For this review, take the finished solid that the model builds, in its own axes (mm). A direction names the side the tool comes from. Coordinates: 2 decimals unless noted, no trailing zeros. Loops run counter-clockwise (first coordinate to the right, second up) from the corner with the lowest first, then second, coordinate; pieces in that order, holes last. Notation, with made-up numbers: (-30.5, 85.5) - (5.5, 85.5) arc R12 cw to (5.5, 101.5) - close; hole circle Ø5 at (63.25, 76). An arc over 180 degrees is marked (long way). One line per item, written item: value. Start each with the question number.
1. Take a section at A-A, the plane z = -383. State the section outline as (x, y) points.
2. Insertion check: pin 1 (3 mm diameter, centred on x = -87, z = 12.5, fed in from +Y); pin 2 (18 mm diameter, centred on y = 21, z = -252.34, fed in from -X); pin 3 (4.5 mm diameter, centred on x = 250, z = 221, fed in from -Y); pin 4 (10 mm diameter, centred on x = 521.5, z = 56.5, fed in from -Y). Each pin has a flat end and moves straight along its axis. Give the tip position at first contact, or say it passes through.
3. The part is to be moulded in two halves that separate along X. For faces 1 (the face through (1351.312, 25, -147)), 2 (the face through (1347.312, 25, -147)), 3 (the face through (385, 25, 222.656)), 4 (the face through (-554.688, 25, -157)), say which applies: released by +X, released by -X, zero draft, split by the parting line, or undercut.
4. To check wall thickness, follow line 1 (Z direction, x = -553.3, y = 21); line 2 (X direction, y = 39, z = -11.5); line 3 (Y direction, x = -222.5, z = -376.5). State the ranges of each line that lie inside material, in increasing order. Write a range as from..to.
5. Take a section at B-B, the plane x = 1007. State the section outline as (y, z) points.
6. For faces 5 (the face through (385, -34, -527.344)), 6 (the face through (-550.688, 25, -157)), 7 (the face through (385, -4, -157)), list the 3-axis set-ups (+Z, -Z, +X, -X, +Y, -Y) from which the entire face can be reached by the end or side of a thin tool; tool diameter is ignored.
```python
from build123d import *

# Parameters (mm, degrees)
SKETCH1_W                    = 1906
SKETCH1_H                    = 750
BASE_FLANGE1_DEPTH           = 4
EDGE_FLANGE1_STRIP_W         = 24
EDGE_FLANGE1_STRIP_H         = 4
EDGE_FLANGE1_STRIP_CUT_DEPTH = 1906
EDGE_FLANGE1_DEPTH           = 1906
EDGE_FLANGE2_STRIP_W         = 24
EDGE_FLANGE2_STRIP_H         = 4
EDGE_FLANGE2_STRIP_CUT_DEPTH = 1906
EDGE_FLANGE2_DEPTH           = 1906
EDGE_FLANGE3_STRIP_W         = 24
EDGE_FLANGE3_STRIP_H         = 4
EDGE_FLANGE3_STRIP_CUT_DEPTH = 734
EDGE_FLANGE3_DEPTH           = 734
EDGE_FLANGE4_STRIP_W         = 24
EDGE_FLANGE4_STRIP_H         = 4
EDGE_FLANGE4_STRIP_CUT_DEPTH = 734
EDGE_FLANGE4_DEPTH           = 734
SKETCH18_R                   = 7
CUT_EXTRUDE4_DEPTH           = 1979.516472174
LPATTERN1_COUNT              = 4
LPATTERN1_PITCH              = 200
CUT_EXTRUDE5_DEPTH           = 10
LPATTERN2_COUNT              = 6
LPATTERN2_PITCH              = 300
CUT_EXTRUDE6_DEPTH           = 1545.720516034
LPATTERN3_COUNT              = 6
LPATTERN3_PITCH              = 300


# Sheet-metal steps are written as plain solids
with BuildPart() as part:
    # Sketch1 → Base-Flange1 (new body)
    with BuildSketch(Plane(origin=(0, 0, 0), x_dir=(1, 0, 0), z_dir=(0, 1, 0))):
        with Locations((398.3125, 152.34375)):
            Rectangle(SKETCH1_W, SKETCH1_H)
    extrude(amount=-BASE_FLANGE1_DEPTH)

    # Edge-Flange1 strip (across the edge) → Edge-Flange1 strip cut (cut)
    with BuildSketch(Plane(origin=(-554.6875, -4, -527.34375), x_dir=(0, 0, 1), z_dir=(1, 0, 0))):
        with Locations((-4, -2)):
            Rectangle(EDGE_FLANGE1_STRIP_W, EDGE_FLANGE1_STRIP_H)
    extrude(amount=EDGE_FLANGE1_STRIP_CUT_DEPTH, mode=Mode.SUBTRACT)

    # Edge-Flange1 section (across the edge) → Edge-Flange1 (add)
    with BuildSketch(Plane(origin=(-554.6875, -4, -527.34375), x_dir=(0, 0, 1), z_dir=(1, 0, 0))):
        with BuildLine():
            Line((0, 4), (0, 56))
            Line((0, 56), (4, 56))
            Line((4, 56), (4, 4))
            ThreePointArc((4, 4), (5.171572875, 1.171572875), (8, 0))
            Line((8, 0), (8, -4))
            ThreePointArc((8, -4), (2.343145751, -1.656854249), (0, 4))
        make_face()
    extrude(amount=EDGE_FLANGE1_DEPTH)

    # Edge-Flange2 strip (across the edge) → Edge-Flange2 strip cut (cut)
    with BuildSketch(Plane(origin=(-554.6875, 0, 222.65625), x_dir=(0, 0, -1), z_dir=(1, 0, 0))):
        with Locations((-4, -2)):
            Rectangle(EDGE_FLANGE2_STRIP_W, EDGE_FLANGE2_STRIP_H)
    extrude(amount=EDGE_FLANGE2_STRIP_CUT_DEPTH, mode=Mode.SUBTRACT)

    # Edge-Flange2 section (across the edge) → Edge-Flange2 (add)
    with BuildSketch(Plane(origin=(-554.6875, 0, 222.65625), x_dir=(0, 0, -1), z_dir=(1, 0, 0))):
        with BuildLine():
            Line((0, 4), (0, 46))
            Line((0, 46), (4, 46))
            Line((4, 46), (4, 4))
            ThreePointArc((4, 4), (5.171572875, 1.171572875), (8, 0))
            Line((8, 0), (8, -4))
            ThreePointArc((8, -4), (2.343145751, -1.656854249), (0, 4))
        make_face()
    extrude(amount=EDGE_FLANGE2_DEPTH)

    # Edge-Flange3 strip (across the edge) → Edge-Flange3 strip cut (cut)
    with BuildSketch(Plane(origin=(1351.3125, 0, 214.65625), x_dir=(-1, 0, 0), z_dir=(0, 0, -1))):
        with Locations((-4, -2)):
            Rectangle(EDGE_FLANGE3_STRIP_W, EDGE_FLANGE3_STRIP_H)
    extrude(amount=EDGE_FLANGE3_STRIP_CUT_DEPTH, mode=Mode.SUBTRACT)

    # Edge-Flange3 section (across the edge) → Edge-Flange3 (add)
    with BuildSketch(Plane(origin=(1351.3125, 0, 214.65625), x_dir=(-1, 0, 0), z_dir=(0, 0, -1))):
        with BuildLine():
            Line((0, 4), (0, 46))
            Line((0, 46), (4, 46))
            Line((4, 46), (4, 4))
            ThreePointArc((4, 4), (5.171572875, 1.171572875), (8, 0))
            Line((8, 0), (8, -4))
            ThreePointArc((8, -4), (2.343145751, -1.656854249), (0, 4))
        make_face()
    extrude(amount=EDGE_FLANGE3_DEPTH)

    # Edge-Flange4 strip (across the edge) → Edge-Flange4 strip cut (cut)
    with BuildSketch(Plane(origin=(-554.6875, 0, -519.34375), x_dir=(1, 0, 0), z_dir=(0, 0, 1))):
        with Locations((-4, -2)):
            Rectangle(EDGE_FLANGE4_STRIP_W, EDGE_FLANGE4_STRIP_H)
    extrude(amount=EDGE_FLANGE4_STRIP_CUT_DEPTH, mode=Mode.SUBTRACT)

    # Edge-Flange4 section (across the edge) → Edge-Flange4 (add)
    with BuildSketch(Plane(origin=(-554.6875, 0, -519.34375), x_dir=(1, 0, 0), z_dir=(0, 0, 1))):
        with BuildLine():
            Line((0, 4), (0, 46))
            Line((0, 46), (4, 46))
            Line((4, 46), (4, 4))
            ThreePointArc((4, 4), (5.171572875, 1.171572875), (8, 0))
            Line((8, 0), (8, -4))
            ThreePointArc((8, -4), (2.343145751, -1.656854249), (0, 4))
        make_face()
    extrude(amount=EDGE_FLANGE4_DEPTH)

    # Sketch18 → Cut-Extrude4 (cut, symmetric)
    with BuildSketch(Plane(origin=(1351.3125, 0, 0), x_dir=(0, 0, -1), z_dir=(1, 0, 0))):
        with Locations(Location((-147.65625, 21, 0), (0, 0, 90))):
            Circle(SKETCH18_R)
    cut_extrude4 = extrude(amount=CUT_EXTRUDE4_DEPTH, both=True, mode=Mode.SUBTRACT)

    # LPattern1: Cut-Extrude4 ×4
    with Locations(*[(0, 0, -i * LPATTERN1_PITCH) for i in range(1, LPATTERN1_COUNT)]):
        add(cut_extrude4, mode=Mode.SUBTRACT)

    # Sketch19 → Cut-Extrude5 (cut)
    with BuildSketch(Plane.XY.offset(222.65625)):
        with BuildLine():
            Line((1153.3125, 14), (1143.3125, 14))
            ThreePointArc((1143.3125, 14), (1136.3125, 21), (1143.3125, 28))
            Line((1143.3125, 28), (1153.3125, 28))
            ThreePointArc((1153.3125, 28), (1160.3125, 21), (1153.3125, 14))
        make_face()
    cut_extrude5 = extrude(amount=-CUT_EXTRUDE5_DEPTH, mode=Mode.SUBTRACT)

    # LPattern2: Cut-Extrude5 ×6
    with Locations(*[(-i * LPATTERN2_PITCH, 0, 0) for i in range(1, LPATTERN2_COUNT)]):
        add(cut_extrude5, mode=Mode.SUBTRACT)

    # Sketch20 → Cut-Extrude6 (cut, symmetric)
    with BuildSketch(Plane.XY.offset(-523.34375)):
        with BuildLine():
            Line((-351.6875, -28), (-341.6875, -28))
            ThreePointArc((-341.6875, -28), (-334.6875, -35), (-341.6875, -42))
            Line((-341.6875, -42), (-351.6875, -42))
            ThreePointArc((-351.6875, -42), (-358.6875, -35), (-351.6875, -28))
        make_face()
    cut_extrude6 = extrude(amount=CUT_EXTRUDE6_DEPTH, both=True, mode=Mode.SUBTRACT)

    # LPattern3: Cut-Extrude6 ×6
    with Locations(*[(i * LPATTERN3_PITCH, 0, 0) for i in range(1, LPATTERN3_COUNT)]):
        add(cut_extrude6, mode=Mode.SUBTRACT)


solid = part.part
```
Solutions:
1. outline: (-554.69, 4) arc R8 ccw to (-546.69, -4) - (1343.31, -4) arc R8 ccw to (1351.31, 4) - (1351.31, 46) - (1347.31, 46) - (1347.31, 4) arc R4 cw to (1343.31, 0) - (-546.69, 0) arc R4 cw to (-550.69, 4) - (-550.69, 46) - (-554.69, 46) - close
2. pin 1: y = 0
2. pin 2: x = -554.69
2. pin 3: y = -2.87
2. pin 4: y = -4
3. face 1: released by +X
3. face 2: undercut
3. face 3: zero draft
3. face 4: released by -X
4. line 1: -519.34..-459.34, -445.34..-259.34, -245.34..-59.34, -45.34..140.66, 154.66..214.66, 218.66..222.66
4. line 2: -554.69..-550.69, 1347.31..1351.31
4. line 3: -4..0
5. outline: (-60, -527.34) - (-8, -527.34) arc R8 ccw to (0, -519.34) - (0, 214.66) arc R4 cw to (4, 218.66) - (46, 218.66) - (46, 222.66) - (4, 222.66) arc R8 ccw to (-4, 214.66) - (-4, -519.34) arc R4 cw to (-8, -523.34) - (-60, -523.34) - close
6. face 5: -Z, +X, -X, +Y, -Y
6. face 6: -Z, +Y
6. face 7: +Z, +X, -X, -Y
